Part model, mm, in its own coordinate system. Face numbers are marked on the shaded views. A direction names the side the tool comes from. Round coordinates to 2 decimals unless told otherwise and drop trailing zeros. Loops run counter-clockwise (first coordinate to the right, second up) from the corner with the lowest first, then second, coordinate; pieces in that order, holes last. Notation, with made-up numbers: (7, 71) -> (52, 71) arc R21 ccw to (52, 75) -> close; hole circle Ø6 at (-4, 85.5). An arc over 180 degrees is marked (long way). Use a Markdown table: item, result. Add a question column.
Item 1: Flat gauge pins, fed straight in: pin 1 (1.5 mm diameter, centred on y = 50, z = 8.5, fed in from -X); pin 2 (9.5 mm diameter, centred on x = 13.5, y = 51.5, fed in from +Z); pin 3 (1.5 mm diameter, centred on x = 13, y = 50.5, fed in from -Z); pin 4 (2.5 mm diameter, centred on x = 19.62, y = 62.38, fed in from +Z). Where does each tip first touch, or does it go through?
Item 2: Two-plate mould, pull along Y, no slides. Class the marked faces 1, 2, 3 and 4: pulls with the +Y half, pulls with the -Y half, needs draft (parallel to the pull), parting line crosses it, or undercut.
Item 3: Which spindle directions (+Z, -Z, +X, -X, +Y, -Y) get a long thin tool onto all of the face, cutting with end or side? Do the marked faces 5, 6 and 7. Say none if no direction does.
Item 4: Cut at C-C, the plane z = -6.5. List the corners of the cut face in (x, y).
Item 5: Cut at A-A, the plane z = -1.5. List the corners of the cut face in (x, y).
Item 6: Probe line 1 (X direction, y = 56.25, z = -3); line 2 (X direction, y = 55, z = 13); line 3 (Z direction, x = 11.5, y = 54.5). List the from-to ranges inside material, lowest first. Write a range as [from, to].
Item 7: Cut at B-B, the plane z = 2.5. State how many separate pieces and enclosed holes the cut face has, plus the area to 3 significant figures.
```python
from build123d import *

# Parameters (mm, degrees)
MODEL_R             = 1.48
MODEL_R_2           = 1.5
BOSS_EXTRUDE1_DEPTH = 12
SKETCH3_W           = 12
SKETCH3_H           = 15.317128206
BOSS_EXTRUDE2_DEPTH = 1.5
BOSS_EXTRUDE3_DEPTH = 1.5
BOSS_EXTRUDE4_START = -4.5
BOSS_EXTRUDE4_DEPTH = 6.26
CHAMFER1_SIZE       = 2.5
FILLET2_R           = 0.5
CUT_EXTRUDE1_DEPTH  = 1


with BuildPart() as part:
    # Model → Boss-Extrude1 (new body)
    with BuildSketch(Plane.XY):
        Polygon((5.6444, 52.0867), (5.2748, 51.5489), (5.0569, 50.9337), (5.0057, 50.2831), (5.1246, 49.6414), (5.4056, 49.0523), (5.8295, 48.556), (7.3157, 47.2178), (7.9717, 46.7918), (8.7273, 46.5893), (9.5084, 46.6303), (10.2386, 46.9106), (10.8464, 47.4028), (22.8908, 60.7794), (23.2604, 61.3173), (23.4783, 61.9325), (23.5295, 62.5831), (23.4106, 63.2248), (23.1296, 63.8138), (22.7058, 64.3101), (21.2195, 65.6484), (20.6816, 66.018), (20.0664, 66.2359), (19.4158, 66.2871), (18.7741, 66.1681), (18.185, 65.8872), (17.6888, 65.4633), align=None)
        with Locations((19.6206, 62.3782)):
            Circle(MODEL_R, mode=Mode.SUBTRACT)
        with Locations((8.9146, 50.4879)):
            Circle(MODEL_R_2, mode=Mode.SUBTRACT)
    extrude(amount=BOSS_EXTRUDE1_DEPTH)

    # Sketch3 → Boss-Extrude2 (add)
    with BuildSketch(Plane(origin=(-22.783506803, 20.514455792, 0), x_dir=(0, 0, 1), z_dir=(-0.743143299, 0.669132302, 0))):
        with Locations((6, 51.484746303)):
            Rectangle(SKETCH3_W, SKETCH3_H)
    extrude(amount=BOSS_EXTRUDE2_DEPTH)

    # Sketch4 → Boss-Extrude3 (add)
    with BuildSketch(Plane(origin=(-23.898221752, 21.518154244, 0), x_dir=(0, 0, 1), z_dir=(-0.743143299, 0.669132302, 0))):
        Polygon((-10.680029898, 56.112643872), (-10.680029898, 59.112643872), (-7.680029898, 59.112643872), (19.680029898, 59.112643872), (22.680029898, 59.112643872), (22.680029898, 56.112643872), (22.680029898, 46.856848734), (22.680029898, 43.856848734), (19.680029898, 43.856848734), (-7.680029898, 43.856848734), (-10.680029898, 43.856848734), (-10.680029898, 46.856848734), align=None)
    extrude(amount=BOSS_EXTRUDE3_DEPTH)

    # Sketch9 → Boss-Extrude4 (add)
    with BuildSketch(Plane(origin=(29.346034145, 32.591923246, 0), x_dir=(0.743143299, -0.669132302, 0), z_dir=(-0.669132302, -0.743143299, 0)).offset(BOSS_EXTRUDE4_START)):
        Polygon((-32.15829543, 12), (-32.15829543, 22.680029898), (-27.158287979, 12), align=None)
    boss_extrude4 = extrude(amount=-BOSS_EXTRUDE4_DEPTH)

    # Mirror1: Boss-Extrude4 across plane
    add(boss_extrude4.mirror(Plane.XY.offset(6)))

    # Chamfer1
    chamfer1_edges = [part.edges().sort_by_distance(p)[0] for p in [
        (15.098600236, 65.949168642, 22.680029898),
        (15.098600236, 65.949168642, -10.680029898),
        (4.890454919, 54.611926717, -10.680029898),
        (4.890454919, 54.611926717, 22.680029898),
    ]]
    chamfer(chamfer1_edges, length=CHAMFER1_SIZE)

    # Fillet2
    fillet2_edges = [part.edges().sort_by_distance(p)[0] for p in [
        (9.437170103, 60.782396906, 22.680029898),
        (4.333097445, 55.113775943, 6),
        (14.541242762, 66.451017868, 6),
        (9.437170103, 60.782396906, -10.680029898),
        (13.704827384, 65.522088744, 21.430029898),
        (13.704827384, 65.522088744, -9.430029898),
        (5.169512823, 56.042705067, -9.430029898),
        (5.169512823, 56.042705067, 21.430029898),
    ]]
    fillet(fillet2_edges, radius=FILLET2_R)

    # Sketch10 → Cut-Extrude1 (cut)
    with BuildSketch(Plane(origin=(-25.0129367, 22.521852697, 0), x_dir=(0, 0, 1), z_dir=(-0.743143299, 0.669132302, 0))):
        with BuildLine():
            Line((19, 53.048695087), (-7, 53.048695087))
            ThreePointArc((-7, 53.048695087), (-9, 55.048695087), (-7, 57.048695087))
            Line((-7, 57.048695087), (19, 57.048695087))
            ThreePointArc((19, 57.048695087), (21, 55.048695087), (19, 53.048695087))
        make_face()
        with BuildLine():
            Line((19, 49.920797519), (-7, 49.920797519))
            ThreePointArc((-7, 49.920797519), (-9, 47.920797519), (-7, 45.920797519))
            Line((-7, 45.920797519), (19, 45.920797519))
            ThreePointArc((19, 45.920797519), (21, 47.920797519), (19, 49.920797519))
        make_face()
    extrude(amount=-CUT_EXTRUDE1_DEPTH, mode=Mode.SUBTRACT)


solid = part.part
```
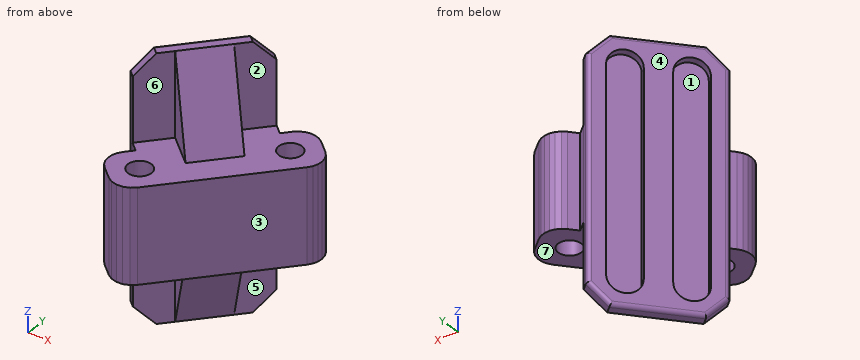
A:
| question | item | result |
|---|---|---|
| 1 | pin 1 | stops at x = 5.01 |
| 1 | pin 2 | stops at z = 16.06 |
| 1 | pin 3 | stops at z = 0 |
| 1 | pin 4 | passes through |
| 2 | face 1 | undercut |
| 2 | face 2 | undercut |
| 2 | face 3 | pulls with the -Y half |
| 2 | face 4 | pulls with the +Y half |
| 3 | face 5 | -Z, +X |
| 3 | face 6 | +Z, -Y |
| 3 | face 7 | -Z |
| 4 | outline | (4.67, 55.49) arc R0.5 ccw to (4.7, 54.78) -> (5.45, 54.11) -> (8.46, 57.45) -> (9.91, 56.14) -> (14.1, 60.8) -> (12.65, 62.11) -> (15.66, 65.45) -> (14.91, 66.12) arc R0.5 ccw to (14.21, 66.08) -> (13.16, 64.92) -> (13.9, 64.25) -> (11.23, 61.28) -> (10.48, 61.94) -> (8.39, 59.62) -> (9.13, 58.95) -> (6.46, 55.98) -> (5.71, 56.65) -> close |
| 5 | outline | (4.67, 55.49) arc R0.5 ccw to (4.7, 54.78) -> (5.45, 54.11) -> (8.46, 57.45) -> (11.65, 54.58) -> (15.84, 59.23) -> (12.65, 62.11) -> (15.66, 65.45) -> (14.91, 66.12) arc R0.5 ccw to (14.21, 66.08) -> (13.16, 64.92) -> (13.9, 64.25) -> (11.23, 61.28) -> (10.48, 61.94) -> (8.39, 59.62) -> (9.13, 58.95) -> (6.46, 55.98) -> (5.71, 56.65) -> close |
| 6 | line 1 | x = [5.36, 6.16], [6.7, 7.37], [9.8, 12.21] |
| 6 | line 2 | x = [4.56, 6.25], [11.18, 12.35] |
| 6 | line 3 | z = [0, 12] |
| 7 | separate pieces | 1 |
| 7 | enclosed holes | 2 |
| 7 | area | 179 mm^2 |
